from build123d import *

# Parameters (mm, degrees)
SKETCH_1_R          = 9
EXTRUDE_1_DEPTH     = 1
SKETCH_2_R          = 6
EXTRUDE_2_DEPTH     = 6.5
SKETCH_3_R          = 0.65
CUT_EXTRUDE_1_DEPTH = 6.5
SKETCH_5_R          = 9
EXTRUDE_3_DEPTH     = 1
SKETCH_6_R          = 1.5
CUT_EXTRUDE_2_DEPTH = 16.305227865


with BuildPart() as part:
    # 草图1 → 凸台-拉伸1 (new body)
    with BuildSketch(Plane(origin=(0, 0, 0), x_dir=(1, 0, 0), z_dir=(0, 1, 0))):
        with Locations(Location((0, 0, 0), (0, 0, 270))):
            Circle(SKETCH_1_R)
    extrude(amount=EXTRUDE_1_DEPTH)

    # 草图2 → 凸台-拉伸2 (add)
    with BuildSketch(Plane(origin=(0, 1, 0), x_dir=(1, 0, 0), z_dir=(0, 1, 0))):
        with Locations(Location((0, 0, 0), (0, 0, 90))):
            Circle(SKETCH_2_R)
    extrude(amount=EXTRUDE_2_DEPTH)

    # 草图3 → 切除-拉伸1 (cut)
    with BuildSketch(Plane(origin=(0, 7.5, 0), x_dir=(1, 0, 0), z_dir=(0, 1, 0))):
        with Locations((0, 6)):
            Circle(SKETCH_3_R)
        with Locations((1.854101966, 5.706339098)):
            Circle(SKETCH_3_R)
        with Locations((3.526711514, 4.854101966)):
            Circle(SKETCH_3_R)
        with Locations((4.854101966, 3.526711514)):
            Circle(SKETCH_3_R)
        with Locations((5.706339098, 1.854101966)):
            Circle(SKETCH_3_R)
        with Locations((6, 0)):
            Circle(SKETCH_3_R)
        with Locations((5.706339098, -1.854101966)):
            Circle(SKETCH_3_R)
        with Locations((4.854101966, -3.526711514)):
            Circle(SKETCH_3_R)
        with Locations((3.526711514, -4.854101966)):
            Circle(SKETCH_3_R)
        with Locations((1.854101966, -5.706339098)):
            Circle(SKETCH_3_R)
        with Locations((0, -6)):
            Circle(SKETCH_3_R)
        with Locations((-1.854101966, -5.706339098)):
            Circle(SKETCH_3_R)
        with Locations((-3.526711514, -4.854101966)):
            Circle(SKETCH_3_R)
        with Locations((-4.854101966, -3.526711514)):
            Circle(SKETCH_3_R)
        with Locations((-5.706339098, -1.854101966)):
            Circle(SKETCH_3_R)
        with Locations((-6, 0)):
            Circle(SKETCH_3_R)
        with Locations((-5.706339098, 1.854101966)):
            Circle(SKETCH_3_R)
        with Locations((-4.854101966, 3.526711514)):
            Circle(SKETCH_3_R)
        with Locations((-3.526711514, 4.854101966)):
            Circle(SKETCH_3_R)
        with Locations((-1.854101966, 5.706339098)):
            Circle(SKETCH_3_R)
    extrude(amount=-CUT_EXTRUDE_1_DEPTH, mode=Mode.SUBTRACT)

    # 草图5 → 凸台-拉伸3 (add)
    with BuildSketch(Plane(origin=(0, 7.5, 0), x_dir=(1, 0, 0), z_dir=(0, 1, 0))):
        with Locations(Location((0, 0, 0), (0, 0, 270))):
            Circle(SKETCH_5_R)
    extrude(amount=EXTRUDE_3_DEPTH)

    # 草图6 → 切除-拉伸2 (cut, through all)
    with BuildSketch(Plane(origin=(0, 8.5, 0), x_dir=(1, 0, 0), z_dir=(0, 1, 0))):
        with Locations(Location((0, 0, 0), (0, 0, 270))):
            Circle(SKETCH_6_R)
    extrude(amount=-CUT_EXTRUDE_2_DEPTH, mode=Mode.SUBTRACT)


solid = part.part
The listing builds one solid part. Answer for the finished solid, in the listing's coordinates (mm). A direction names the side the tool comes from. Give positions to 0.01 mm unless a question says otherwise; leave off trailing zeros. Write each loop counter-clockwise with the first axis right and the second up, starting at its lowest first coordinate (ties: lowest second). Pieces come first, ordered by that corner, then holes. Notation, with made-up numbers: (-11.75, 51) -> (19.25, 51) arc R33 ccw to (19.25, 86) -> close; hole circle Ø8 at (-37, 7). An arc over 180 degrees is marked (long way). Use a Markdown table: item, result.
(1) Section D-D, the plane z = 0 is taken. Determine the outline of the cut face in (x, y).
Return value:
| item | result |
|---|---|
| outline | (-9, 0) -> (-1.5, 0) -> (-1.5, 8.5) -> (-9, 8.5) -> (-9, 7.5) -> (-5.35, 7.5) -> (-5.35, 1) -> (-9, 1) -> close; (1.5, 0) -> (9, 0) -> (9, 1) -> (5.35, 1) -> (5.35, 7.5) -> (9, 7.5) -> (9, 8.5) -> (1.5, 8.5) -> close |
(2) Section A-A, the plane x = 0 is taken. Determine the outline of the cut face in (y, z), then the cut area to 4 significant figures.
Return value:
| item | result |
|---|---|
| outline | (0, -9) -> (1, -9) -> (1, -5.35) -> (7.5, -5.35) -> (7.5, -9) -> (8.5, -9) -> (8.5, -1.5) -> (0, -1.5) -> close; (0, 1.5) -> (8.5, 1.5) -> (8.5, 9) -> (7.5, 9) -> (7.5, 5.35) -> (1, 5.35) -> (1, 9) -> (0, 9) -> close |
| area | 80.05 mm2 |
(3) Find the intervals of material crossed by probe 1 along X at (y, z) = (4.75, 0); probe 2 along Y at (x, z) = (1.5, 7); probe 3 along Z at (x, y) = (5.25, 4), in increasing order. Write a range as from..to.
Return value:
| item | result |
|---|---|
| probe 1 | -5.35..-1.5, 1.5..5.35 |
| probe 2 | 0..1, 7.5..8.5 |
| probe 3 | -2.9..-2.32, -1.39..1.39, 2.32..2.9 |
(4) Section C-C, the plane y = 8.25 is taken. Determine the outline of the cut face in (x, z).
Return value:
| item | result |
|---|---|
| outline | circle Ø18 at (0, 0); hole circle Ø3 at (0, 0) |
(5) Flat-ended cylindrical pins translate along their axes: P1, Ø2, axis at x = 0.5, y = 4, coming from the -Z side; P2, Ø2, axis at y = 3, z = 6, coming from the +X side; P3, Ø3, axis at y = 4.5, z = 5.5, coming from the -X side. Find the tip coordinate at first contact, or state that the pin passes through.
Return value:
| item | result |
|---|---|
| P1 | z = -5.96 |
| P2 | x = 2.98 |
| P3 | x = -4.44 |
(6) For faces 5 (the cylindrical face through (-5.093, 4.296, -1.64)), 6 (the cylindrical face through (0.45, 4.31, 1.43)), determine the directions among +Z, -Z, +X, -X, +Y, -Y from which every point of the face is accessible in a straight line to the end or side of a thin tool.
Return value:
| item | result |
|---|---|
| face 5 | none |
| face 6 | +Y, -Y |
(7) Section B-B, the plane z = -6.25 is taken. Determine the outline of the cut face in (x, y).
Return value:
| item | result |
|---|---|
| outline | (-6.48, 0) -> (6.48, 0) -> (6.48, 1) -> (-6.48, 1) -> close; (-6.48, 7.5) -> (6.48, 7.5) -> (6.48, 8.5) -> (-6.48, 8.5) -> close |
(8) Determine the mould class of faces 1 (the cylindrical face through (3.13, 4.3, -4.34)), 2 (the cylindrical face through (5.35, 4.3, -0.01)), 3 (the cylindrical face through (0.01, 4.3, 5.35)), 4 (the flat face through (-2, 0, 0)) for opening direction X: released by +X, released by -X, zero draft, split by the parting line, or undercut.
Return value:
| item | result |
|---|---|
| face 1 | undercut |
| face 2 | released by +X |
| face 3 | undercut |
| face 4 | zero draft |
